```python
from build123d import *

# Parameters (mm, degrees)
F0_R     = 10
F1_DEPTH = 25
F2_R     = 5.5
F3_DEPTH = 10
F4_SIZE  = 2


# Not quite as in the source:
# - a fillet or chamfer that OpenCascade refuses, or shapes differently, is made with other operations: its cross-section is extruded or revolved along the edge and cut away or added


with BuildPart() as f1:
    # F0 (on Front) → F1 (new body)
    with BuildSketch(Plane.XZ):
        Circle(F0_R)
    extrude(amount=F1_DEPTH)

    # F2 (on face) → F3 (cut)
    with BuildSketch(Plane.XZ.offset(25)):
        Circle(F2_R)
    extrude(amount=-F3_DEPTH, mode=Mode.SUBTRACT)

    # F4
    f4_edges = [f1.edges().sort_by_distance(p)[0] for p in [
        (-10, 0, 0),
    ]]
    chamfer(f4_edges, length=F4_SIZE)

    # F5: chamfer of 5 on 1 edges, made by hand

    # F5_s1 → F5_t2 (revolve, cut)
    with BuildSketch(Plane.XY):
        Polygon((10, -20), (5, -25), (10, -25), align=None)
    revolve(axis=Axis((0, -25, 0), (0, -1, 0)), mode=Mode.SUBTRACT)


solid = f1.part
```
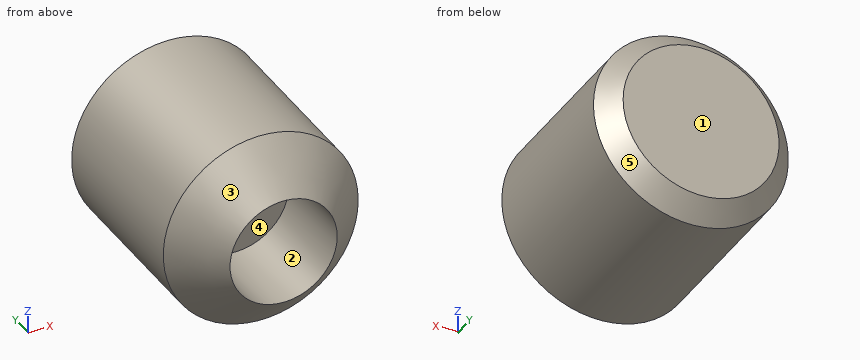
Part model, mm, in its own coordinate system. Face numbers are marked on the shaded views. A direction names the side the tool comes from. Give positions to 0.01 mm unless a question says otherwise; leave off trailing zeros. Write each loop counter-clockwise with the first axis right and the second up, starting at its lowest first coordinate (ties: lowest second). Pieces come first, ordered by that corner, then holes. Notation, with made-up numbers: (5, 18) -> (18, 18) arc R25 ccw to (18, 30) -> close; hole circle Ø6 at (-10.5, 42). An arc over 180 degrees is marked (long way). Put each result on its own line as item: value. Start each with the question number.
Item 1: Pull direction X, two halves, no side cores. Call the marked faces 1, 2 and 3: pulls with the +X half, pulls with the -X half, needs draft (parallel to the pull), parting line crosses it, or undercut.
Item 2: Pin check, flat tips, straight feed: pin 1 Ø6 at (y, z) = (-10.5, 1) entering from -X; pin 2 Ø2 at (y, z) = (-3, 3.5) entering from +X; pin 3 Ø1 at (y, z) = (-15, -6) entering from -X; pin 4 Ø1.5 at (x, y) = (5.5, -18) entering from -Z. Stop position of each tip, or through.
Item 3: Cut at A-A (x = 0). List the corners of the cut face in (y, z).
Item 4: Cut at B-B (z = 0). List the corners of the cut face in (x, y), then the cut area to 3 significant figures.
Item 5: Cut at C-C (y = -7.25). List the corners of the cut face in (x, z), then the cut area to 3 significant figures.
Item 6: Which spindle directions (+Z, -Z, +X, -X, +Y, -Y) get a long thin tool onto all of the face, cutting with end or side? Do the marked faces 4 and 5. Say none if no direction does.
Item 7: Wall check: L1, parallel to Z at x = 0, y = -17; L2, parallel to Y at x = -1.25, z = -5.25; L3, parallel to X at y = -15.75, z = -6. Give the ranges that are in metal, low to high. Write a range as [from, to].
Answer list:
1. face 1: needs draft
1. face 2: undercut
1. face 3: parting line crosses it
2. pin 1: stops at x = -10
2. pin 2: stops at x = 9.68
2. pin 3: stops at x = -8.35
2. pin 4: stops at z = -8.8
3. outline: (-24.5, -5.5) -> (-20, -10) -> (-2, -10) -> (0, -8) -> (0, 8) -> (-2, 10) -> (-20, 10) -> (-24.5, 5.5) -> (-15, 5.5) -> (-15, -5.5) -> close
4. outline: (-10, -20) -> (-5.5, -24.5) -> (-5.5, -15) -> (5.5, -15) -> (5.5, -24.5) -> (10, -20) -> (10, -2) -> (8, 0) -> (-8, 0) -> (-10, -2) -> close
4. area: 361 mm2
5. outline: circle Ø20 at (0, 0)
5. area: 314 mm2
6. face 4: -Y
6. face 5: +Y
7. L1: z = [-10, -5.5], [5.5, 10]
7. L2: y = [-15, 0]
7. L3: x = [-8, 8]
